Here's the drawing with two shaded views (mm, measured from the low corner). I have some questions. A direction names the side the tool comes from. Round coordinates to 2 decimals unless told otherwise and drop trailing zeros. Write each loop counter-clockwise with the first axis right and the second up, starting at its lowest first coordinate (ties: lowest second). Pieces come first, ordered by that corner, then holes. Notation, with made-up numbers: M -25.75,79 L 11.25,79 A18 cw 11.25,105 Z; hole C -34.5,19 d7. An arc over 180 degrees is marked long. Answer as a JSON object with one key per item and string values. Group by question number.
1) On a 3-axis mill with a long thin cutter (end or side, diameter ignored), from which of +Z, -Z, +X, -X, +Y, -Y can I reach the whole of each face in a straight line? I mean the marked faces 4, 5 and 6. Say none if no direction works.
2) If we mould it in two halves opening along Y, with no side actions, what happens to the marked faces 1, 2 and 3? For each: +Y half, -Y half, draft (parallel to the pull), parting line (faces both ways), or undercut.
3) Suppose I cut it at C-C, the plane y = 7.5. Write out the boundary of the cut face in (x, z).
4) I'm going to push flat-ended pins straight in: pin 1 Ø1.2 at (x, z) = (22.5, 6) entering from -Y; pin 2 Ø1.5 at (x, z) = (15, 8) entering from +Y. Where does each tip first touch, or does it pass through?
5) Please list where these lines run through material, in increasing order: L1, parallel to Z at x = 22, y = 8.25; L2, parallel to X at y = 3.5, z = 12.5; L3, parallel to Y at x = 20, z = 9. Write a range as [from, to].
6) Suppose I cut it at D-D, the plane x = 2.5. Write out the boundary of the cut face in (y, z), and give its area (3 significant figures).
7) Suppose I cut it at B-B, the plane z = 9. Write out the boundary of the cut face in (x, y), and give its area (3 significant figures).
8) Suppose I cut it at A-A, the plane y = 28.5. Write out the boundary of the cut face in (x, z), and give its area (3 significant figures).
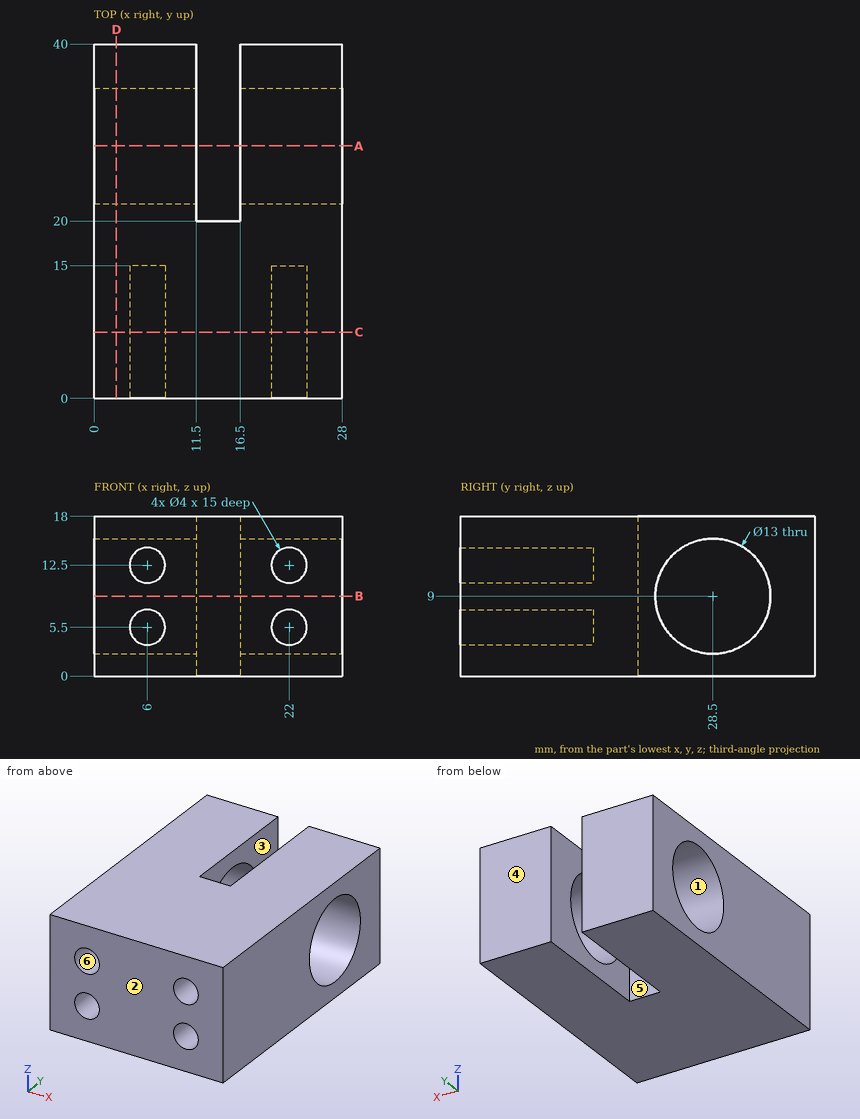
Results:
{
 "1": {"face 4": "+Z, -Z, +X, -X, +Y", "face 5": "+Z, -Z, +Y", "face 6": "-Y"},
 "2": {"face 1": "undercut", "face 2": "-Y half", "face 3": "draft"},
 "3": {"outline": "M 0,0 L 28,0 L 28,18 L 0,18 Z; hole C 6,5.5 d4; hole C 6,12.5 d4; hole C 22,5.5 d4; hole C 22,12.5 d4"},
 "4": {"pin 1": "y = 15", "pin 2": "y = 20"},
 "5": {"L1": "[0, 3.5], [7.5, 10.5], [14.5, 18]", "L2": "[0, 4], [8, 20], [24, 28]", "L3": "[0, 22], [35, 40]"},
 "6": {"outline": "M 0,0 L 40,0 L 40,18 L 0,18 Z; hole C 28.5,9 d13", "area": "587 mm^2"},
 "7": {"outline": "M 0,0 L 28,0 L 28,22 L 16.5,22 L 16.5,20 L 11.5,20 L 11.5,22 L 0,22 Z; M 0,35 L 11.5,35 L 11.5,40 L 0,40 Z; M 16.5,35 L 28,35 L 28,40 L 16.5,40 Z", "area": "721 mm^2"},
 "8": {"outline": "M 0,0 L 11.5,0 L 11.5,2.5 L 0,2.5 Z; M 0,15.5 L 11.5,15.5 L 11.5,18 L 0,18 Z; M 16.5,0 L 28,0 L 28,2.5 L 16.5,2.5 Z; M 16.5,15.5 L 28,15.5 L 28,18 L 16.5,18 Z", "area": "115 mm^2"}
}
